Geometry: final body of the model. Coordinates: model frame, mm. Face numbers are marked on the shaded views. A direction names the side the tool comes from. Give positions to 0.01 mm unless a question says otherwise; leave off trailing zeros. Loops run counter-clockwise (first coordinate to the right, second up) from the corner with the lowest first, then second, coordinate; pieces in that order, holes last. Notation, with made-up numbers: (-8, 39) -> (32, 39) arc R28 cw to (32, 66) -> close; hole circle Ø8 at (46.25, 5.5). An arc over 180 degrees is marked (long way). One line per item, written item: value. Start each with the question number.
from build123d import *

# Parameters (mm, degrees)
SCHIZZO1_W                   = 300
SCHIZZO1_H                   = 120
ESTRUSIONE_ESTRUSIONE1_DEPTH = 10
SCHIZZO4_R                   = 60
ESTRUSIONE_ESTRUSIONE2_DEPTH = 40
SCHIZZO5_R                   = 48
TAGLIO_ESTRUSIONE1_DEPTH     = 46
SCHIZZO6_R                   = 4.25
TAGLIO_ESTRUSIONE2_DEPTH     = 46
SCHIZZO7_W                   = 20
SCHIZZO7_H                   = 2
TAGLIO_ESTRUSIONE3_DEPTH     = 46
FORO_PER_VITE_M3_1_D         = 3.4
FORO_PER_VITE_M3_1_DEPTH     = 5
FORO_PER_VITE_M3_1_TIP       = 1.021463052


with BuildPart() as part:
    # Schizzo1 → Estrusione-Estrusione1 (new body)
    with BuildSketch(Plane(origin=(0, 0, 0), x_dir=(1, 0, 0), z_dir=(0, 1, 0))):
        with Locations((-150, 60)):
            Rectangle(SCHIZZO1_W, SCHIZZO1_H)
    extrude(amount=ESTRUSIONE_ESTRUSIONE1_DEPTH)

    # Schizzo4 → Estrusione-Estrusione2 (add)
    with BuildSketch(Plane(origin=(0, 10, 0), x_dir=(1, 0, 0), z_dir=(0, 1, 0))):
        with Locations(Location((-100, 60, 0), (0, 0, 270))):
            Circle(SCHIZZO4_R)
    extrude(amount=ESTRUSIONE_ESTRUSIONE2_DEPTH)

    # Schizzo5 → Taglio-Estrusione1 (cut)
    with BuildSketch(Plane.XZ):
        with Locations(Location((-100, -60, 0), (0, 0, 270))):
            Circle(SCHIZZO5_R)
    extrude(amount=-TAGLIO_ESTRUSIONE1_DEPTH, mode=Mode.SUBTRACT)

    # Schizzo6 → Taglio-Estrusione2 (cut)
    with BuildSketch(Plane.XZ.offset(-46)):
        with Locations(Location((-100, -60, 0), (0, 0, 270))):
            Circle(SCHIZZO6_R)
    extrude(amount=-TAGLIO_ESTRUSIONE2_DEPTH, mode=Mode.SUBTRACT)

    # Schizzo7 → Taglio-Estrusione3 (cut)
    with BuildSketch(Plane.ZY.offset(160)):
        with Locations((-60, 11)):
            Rectangle(SCHIZZO7_W, SCHIZZO7_H)
    extrude(amount=-TAGLIO_ESTRUSIONE3_DEPTH, mode=Mode.SUBTRACT)

    # Foro per Vite M3-1
    with Locations(Plane(origin=(0, 50, 0), x_dir=(1, 0, 0), z_dir=(0, 1, 0))):
        with Locations((-154, 60), (-100, 114), (-46, 60), (-100, 6)):
            Hole(FORO_PER_VITE_M3_1_D / 2, depth=FORO_PER_VITE_M3_1_DEPTH)
            with Locations((0, 0, -(FORO_PER_VITE_M3_1_DEPTH + FORO_PER_VITE_M3_1_TIP / 2))):  # 118° drill point
                Cone(0, FORO_PER_VITE_M3_1_D / 2, FORO_PER_VITE_M3_1_TIP, mode=Mode.SUBTRACT)


solid = part.part
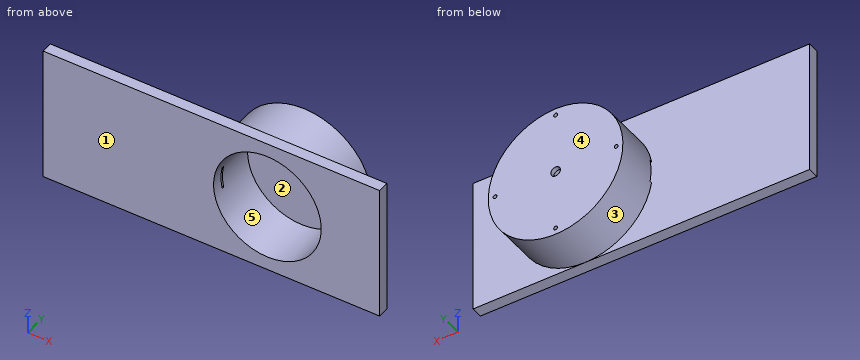
Item 1: Section D-D, the plane x = -138. Output: boundary loops of the cut face in (y, z), then the cut area to 3 significant figures.
Item 2: Pin query (flat end, axial travel): pin 1 (10.5 mm diameter, centred on x = -156.5, z = -57, fed in from -Y); pin 2 (4 mm diameter, centred on y = 19.5, z = -69.5, fed in from -X); pin 3 (3 mm diameter, centred on x = -46, z = -60, fed in from +Y); pin 4 (6 mm diameter, centred on x = -197.5, z = -24.5, fed in from +Y). Return the tip coordinate at first contact, or that it passes through.
Item 3: Section C-C, the plane z = -94. Output: boundary loops of the cut face in (x, y).
Item 4: Access query for the marked faces 4 and 5. Directions: +Z, -Z, +X, -X, +Y, -Y. A direction counts if a zero-diameter tool reaches every point of the face in a straight line with its end or side. Return the directions, or none.
Item 5: Section B-B, the plane x = -184.5. Output: boundary loops of the cut face in (y, z), then the cut area to 3 significant figures.
Item 6: Section A-A, the plane y = 6. Output: boundary loops of the cut face in (x, z), then the cut area to 3 significant figures.
Item 7: Ray query, line 1 along X through (y, z) = (48, -60); line 2 along X through (y, z) = (14, -60); line 3 along Y through (x, z) = (-136, -49). Return the intervals inside material, ascending. Write a range as [from, to].
Item 8: Mould query, pull axis Z, two halves, no side actions, for the marked faces 1, 2 and 3. Classes: pulls with the +Z half, pulls with the -Z half, needs draft (parallel to the pull), parting line crosses it, or undercut.
Geometry check:
1. outline: (0, -120) -> (10, -120) -> (10, -106.43) -> (50, -106.43) -> (50, -13.57) -> (10, -13.57) -> (10, 0) -> (0, 0) -> (0, -30.67) -> (46, -30.67) -> (46, -89.33) -> (0, -89.33) -> close
1. area: 2,220 mm2
2. pin 1: stops at y = 0
2. pin 2: stops at x = -159.53
2. pin 3: stops at y = 44.88
2. pin 4: stops at y = 10
3. outline: (-300, 0) -> (-133.88, 0) -> (-133.88, 46) -> (-66.12, 46) -> (-66.12, 0) -> (0, 0) -> (0, 10) -> (-50.56, 10) -> (-50.56, 50) -> (-149.44, 50) -> (-149.44, 10) -> (-300, 10) -> close
4. face 4: +Z, -Z, +X, -X, +Y
4. face 5: -Y
5. outline: (0, -120) -> (10, -120) -> (10, 0) -> (0, 0) -> close
5. area: 1,200 mm2
6. outline: (-300, -120) -> (0, -120) -> (0, 0) -> (-300, 0) -> close; hole circle Ø96 at (-100, -60)
6. area: 28,800 mm2
7. line 1: x = [-160, -155.7], [-152.3, -104.25], [-95.75, -47.7], [-44.3, -40]
7. line 2: x = [-160, -148], [-52, -40]
7. line 3: y = [46, 50]
8. face 1: needs draft
8. face 2: undercut
8. face 3: parting line crosses it
